from build123d import *

# Parameters (mm, degrees)
F0_W          = 482.6
F0_H          = 25.4
F1_DEPTH      = 101.6
F2_W          = 482.6
F2_H          = 152.4
F3_DEPTH      = 101.6
F4_R          = 6.35
F5_DEPTH      = 266.701
F5_DEPTH_BACK = 266.701
F6_R          = 6.35
F7_DEPTH      = 25.4


with BuildPart() as f1:
    # F0 (on Front) → F1 (new body)
    with BuildSketch(Plane.XZ):
        Polygon((266.7, 101.6), (-266.7, 101.6), (-266.7, 76.2), (-241.3, 76.2), (241.3, 76.2), (266.7, 76.2), align=None)
        Polygon((-241.3, 76.2), (-266.7, 76.2), (-266.7, -101.6), (-241.3, -101.6), (-241.3, -76.2), align=None)
        Polygon((266.7, -101.6), (266.7, 76.2), (241.3, 76.2), (241.3, -76.2), (241.3, -101.6), align=None)
        with Locations((0, -88.9)):
            Rectangle(F0_W, F0_H)
    extrude(amount=-F1_DEPTH)

    # F2 (on face) → F3 (cut)
    with BuildSketch(Plane.XZ):
        Rectangle(F2_W, F2_H)
    extrude(amount=-F3_DEPTH, mode=Mode.SUBTRACT)

    # F4 (on Right) → F5 (cut, two sides)
    with BuildSketch(Plane.YZ) as f5_sk:
        with Locations((50.8, 0)):
            Circle(F4_R)
    extrude(amount=F5_DEPTH, mode=Mode.SUBTRACT)
    extrude(f5_sk.sketch, amount=-F5_DEPTH_BACK, mode=Mode.SUBTRACT)

    # F6 (on face) → F7 (cut)
    with BuildSketch(Plane.XY.offset(101.6)):
        with Locations((-88.9, 50.8)):
            Circle(F6_R)
        with Locations((88.9, 50.8)):
            Circle(F6_R)
    extrude(amount=-F7_DEPTH, mode=Mode.SUBTRACT)


solid = f1.part
The model under review builds one solid part; all positions refer to its coordinate system, in mm. A direction names the side the tool comes from. Round coordinates to 2 decimals unless told otherwise and drop trailing zeros. Loops run counter-clockwise (first coordinate to the right, second up) from the corner with the lowest first, then second, coordinate; pieces in that order, holes last. Notation, with made-up numbers: (57.25, 1.5) - (71.25, 1.5) arc R12 ccw to (71.25, 22.5) - close; hole circle Ø10 at (60.5, 12.25). An arc over 180 degrees is marked (long way). Use CSV: the item, a comma, the result in double quotes.
(1) For line 1 (X direction, y = 50, z = 96); line 2 (Z direction, x = 148, y = 75); line 3 (X direction, y = 31.5, z = -48), list the stretches that pass through material, from the lowest coordinate up.
Working result:
line 1,"x = -266.7 to -95.2, -82.6 to 82.6, 95.2 to 266.7"
line 2,"z = -101.6 to -76.2, 76.2 to 101.6"
line 3,"x = -266.7 to -241.3, 241.3 to 266.7"
(2) Take a section at C-C, the plane z = 0. Give the boundary of the cut face in (x, y), plus the area to 3 significant figures.
Working result:
outline,"(-266.7, 0) - (-241.3, 0) - (-241.3, 44.45) - (-266.7, 44.45) - close; (-266.7, 57.15) - (-241.3, 57.15) - (-241.3, 101.6) - (-266.7, 101.6) - close; (241.3, 0) - (266.7, 0) - (266.7, 44.45) - (241.3, 44.45) - close; (241.3, 57.15) - (266.7, 57.15) - (266.7, 101.6) - (241.3, 101.6) - close"
area,"4,520 mm^2"
(3) Machinability: for faces 4 (the flat face through (-21, 0, -82)), 5 (the flat face through (-3, 50, 76.2)), 6 (the cylindrical face through (84.22, 55.09, 89.08)), which of the approach directions +Z, -Z, +X, -X, +Y, -Y give a long, thin tool a straight path to every point of the face, cutting with its end or side? Answer none if there is none.
Working result:
face 4,"+Z, -Z, +X, -X, -Y"
face 5,"+Y, -Y"
face 6,"+Z"
(4) Take a section at D-D, the plane x = -23.5. Give the boundary of the cut face in (y, z), plus the area to 3 significant figures.
Working result:
outline,"(0, -101.6) - (101.6, -101.6) - (101.6, -76.2) - (0, -76.2) - close; (0, 76.2) - (101.6, 76.2) - (101.6, 101.6) - (0, 101.6) - close"
area,"5,160 mm^2"
(5) Take a section at A-A, the plane x = -88.9. Give the boundary of the cut face in (y, z), plus the area to 3 significant figures.
Working result:
outline,"(0, -101.6) - (101.6, -101.6) - (101.6, -76.2) - (0, -76.2) - close; (0, 76.2) - (44.45, 76.2) - (44.45, 101.6) - (0, 101.6) - close; (57.15, 76.2) - (101.6, 76.2) - (101.6, 101.6) - (57.15, 101.6) - close"
area,"4,840 mm^2"
(6) The part is to be moulded in two halves that separate along Y. For faces 1 (the flat face through (-241.3, 61, -1)), 2 (the flat face through (-21, 101.6, -82)), 3 (the cylindrical face through (-82.843, 52.707, 89.078)), say which applies: pulls with the +Y half, pulls with the -Y half, needs draft (parallel to the pull), parting line crosses it, or undercut.
Working result:
face 1,"needs draft"
face 2,"pulls with the +Y half"
face 3,"undercut"
(7) Take a section at B-B, the plane y = 28. Give the boundary of the cut face in (x, z), plus the area to 3 significant figures.
Working result:
outline,"(-266.7, -101.6) - (266.7, -101.6) - (266.7, 101.6) - (-266.7, 101.6) - close; hole (-241.3, -76.2) - (241.3, -76.2) - (241.3, 76.2) - (-241.3, 76.2) - close"
area,"34,800 mm^2"
(8) Clearance check with flat-ended pins moving along their axes: P1, Ø20.5, axis at y = 50.8, z = 0, coming from the +X side; P2, Ø7.5, axis at y = 50.8, z = 0, coming from the -X side; P3, Ø11.5, axis at x = -88.9, y = 50.8, coming from the +Z side. State where each tip first meets the part, or that it passes through.
Working result:
P1,"stops at x = 266.7"
P2,"passes through"
P3,"stops at z = -76.2"
